For this review, take the finished solid that the model builds, in its own axes (mm). A direction names the side the tool comes from. Round coordinates to 2 decimals unless told otherwise and drop trailing zeros. Loops run counter-clockwise (first coordinate to the right, second up) from the corner with the lowest first, then second, coordinate; pieces in that order, holes last.
1. Consider section A-A on z = -10. State the section outline as (x, y) points.
2. Draft analysis for pull direction Z (two halves, no side actions). For faces 1 (the flat face through (5, -3, -123.5)), 2 (the flat face through (3.565, 5.255, -44.078)), state which applies: released by +Z, released by -Z, zero draft, split by the parting line, or undercut.
3. Tool access review of faces 3 (the flat face through (-3.565, -5.255, -164.79)), 4 (the cylindrical face through (-6.34, 0.32, -183.01)), 5 (the cylindrical face through (5.435, 0.844, -149.014)): name each direction out of +Z, -Z, +X, -X, +Y, -Y from which nothing blocks a thin tool from reaching the whole face with its end or side.
4. Clearance check with flat-ended pins moving along their axes: pin 1 Ø3 at (y, z) = (4.5, -95) entering from -X; pin 2 Ø1 at (y, z) = (2.5, -140) entering from +X; pin 3 Ø2 at (y, z) = (2, -58.5) entering from -X. State where each tip first meets the part, or that it passes through.
5. To check wall thickness, follow line 1 along X through (y, z) = (-0.5, -99.5); line 2 along X through (y, z) = (1, -14); line 3 along Y through (x, z) = (2.5, -173.5). State the ranges of each line that lie inside material, in increasing order.
Solid Edge part; units mm, degrees
sketch "Sketch1" plane through (0, 0, 0) normal (0, 0, 1) x (1, 0, 0)
  line L0 (-6.1009, 4.0673) -> (-6.5728, -3.2499)
  line L1 (-6.5728, -3.2499) -> (-0.4719, -7.3171)
  line L2 (-0.4719, -7.3171) -> (6.1009, -4.0673)
  line L3 (6.1009, -4.0673) -> (6.5728, 3.2499)
  line L4 (6.5728, 3.2499) -> (0.4719, 7.3171)
  line L5 (0.4719, 7.3171) -> (-6.1009, 4.0673)
extrude "Protrusion1" add sketch "Sketch1" against normal blind 180
sketch "Sketch2" plane through (0, 0, -30) normal (0, 0, 1) x (0.0644, 0.9979, 0)
  circle A0 centre (0, 0) radius 5.5
  circle A1 centre (0, 0) radius 13.1424
extrude "ExtrudedCutout_3" cut sketch "Sketch2" against normal blind 2
sketch "Sketch3" plane through (0, 0, -150) normal (0, 0, -1) x (0.8964, 0.4432, 0)
  circle A0 centre (0, 0) radius 13.1424
  circle A1 centre (0, 0) radius 5.5
extrude "ExtrudedCutout_5" cut sketch "Sketch3" against normal blind 2
sketch "Sketch4" plane through (0, 0, -58.5) normal (0, 0, 1) x (0.0644, 0.9979, 0)
  circle A0 centre (0, 0) radius 5.5
  circle A1 centre (0, 0) radius 13.1424
extrude "ExtrudedCutout_7" cut sketch "Sketch4" along normal blind 2
sketch "Sketch5" plane through (0, 0, -121.5) normal (0, 0, -1) x (-0.0644, -0.9979, 0)
  circle A0 centre (0, 0) radius 5.5
  circle A1 centre (0, 0) radius 13.1424
extrude "ExtrudedCutout_8" cut sketch "Sketch5" along normal blind 2
sketch "Sketch6" plane through (0, 0, -180) normal (0, 0, -1) x (-0.0644, -0.9979, 0)
  line L0 (3.6662, -6.35) -> (-3.6662, -6.35)
  line L1 (-3.6662, -6.35) -> (-7.3323, 0)
  line L2 (-7.3323, 0) -> (-3.6662, 6.35)
  line L3 (-3.6662, 6.35) -> (3.6662, 6.35)
  line L4 (3.6662, 6.35) -> (7.3323, 0)
  line L5 (7.3323, 0) -> (3.6662, -6.35)
extrude "ExtrudedProtrusion_2" add sketch "Sketch6" along normal blind 6
sketch "Sketch7" plane through (0, 0, 0) normal (0, 0, 1) x (1, 0, 0)
  line L0 (-6.1009, 4.0673) -> (-6.5728, -3.2499)
  line L1 (-6.5728, -3.2499) -> (-0.4719, -7.3171)
  line L2 (-0.4719, -7.3171) -> (6.1009, -4.0673)
  line L3 (6.1009, -4.0673) -> (6.5728, 3.2499)
  line L4 (6.5728, 3.2499) -> (0.4719, 7.3171)
  line L5 (0.4719, 7.3171) -> (-6.1009, 4.0673)
extrude "ExtrudedProtrusion_3" add sketch "Sketch7" along normal blind 6
sketch "Sketch8" plane through (0, 0, 4) normal (0, 0, 1) x (-0.8964, -0.4432, 0)
  circle A0 centre (0, 0) radius 6.35
  circle A1 centre (0, 0) radius 13.1424
extrude "ExtrudedCutout_9" cut sketch "Sketch8" against normal blind 2
sketch "Sketch9" plane through (0, 0, -184) normal (0, 0, -1) x (0.8964, 0.4432, 0)
  circle A0 centre (0, 0) radius 6.35
  circle A1 centre (0, 0) radius 13.1424
extrude "ExtrudedCutout_10" cut sketch "Sketch9" against normal blind 2
properties part number "BumbleB0517"
Resolved:
1. outline: (-6.57, -3.25) - (-0.47, -7.32) - (6.1, -4.07) - (6.57, 3.25) - (0.47, 7.32) - (-6.1, 4.07) - close
2. face 1: undercut
2. face 2: zero draft
3. face 3: +Z, -Z, -X, -Y
3. face 4: -X
3. face 5: none
4. pin 1: stops at x = -6.17
4. pin 2: stops at x = 6.56
4. pin 3: stops at x = -6.3
5. line 1: x = -6.4 to 6.33
5. line 2: x = -6.3 to 6.43
5. line 3: y = -5.85 to 5.97
